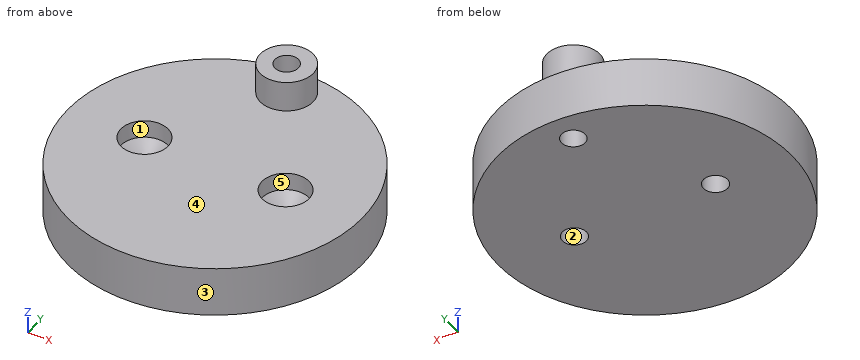
Autodesk Fusion 360 part; units mm, degrees
sketch "Esquisse1" plane through (0, 0, 0) normal (0, 0, 1) x (1, 0, 0)
  circle A0 centre (0, 0) radius 25
  circle A1 centre (-12, 0) radius 2.05
  circle A2 centre (12, 0) radius 2.05
  circle A3 centre (0, 20) radius 2
  dimension "d1" = 50
  dimension "d2" = 4.1
  dimension "d3" = 4.1
  dimension "d4" = 24
  dimension "d5" = 12
  dimension "d6" = 4
  dimension "d7" = 20
extrude "Extrusion1" add sketch "Esquisse1" along normal blind 8.5
sketch "Esquisse2" plane through (0, 0, 8.5) normal (0, 0, 1) x (-1, 0, 0)
  circle A0 centre (0, -20) radius 2
  circle A1 centre (-12, 0) radius 2.05
  circle A2 centre (12, 0) radius 2.05
  circle A3 centre (0, 0) radius 25
  circle A4 centre (0, -20) radius 4.5
  dimension "d10" = 9
extrude "Extrusion2" add sketch "Esquisse2" along normal blind 5.2 contours A4
sketch "Esquisse3" plane through (0, 0, 8.5) normal (0, 0, 1) x (-1, 0, 0)
  circle A0 centre (0, -20) radius 4.5
  circle A1 centre (-12, 0) radius 2.05
  circle A2 centre (12, 0) radius 2.05
  circle A3 centre (0, 0) radius 25
  circle A4 centre (12, 0) radius 4
  circle A5 centre (-12, 0) radius 4
  dimension "d13" = 8
  dimension "d14" = 8
extrude "Extrusion3" cut sketch "Esquisse3" against normal blind 3 contours A4 | A5
hole "Perçage1" at (-12, 0, 5.5) direction (0, 0, -1) diameter 4 depth 10 tip angle 118 countersink diameter 8 countersink angle 90
hole "Perçage2" at (12, 0, 5.5) direction (0, 0, -1) diameter 4 depth 10 tip angle 118 countersink diameter 8 countersink angle 90
The listing builds one solid part. Answer for the finished solid, in the listing's coordinates (mm). Face numbers are marked on the shaded views. A direction names the side the tool comes from. Round coordinates to 2 decimals unless told otherwise and drop trailing zeros. Write each loop counter-clockwise with the first axis right and the second up, starting at its lowest first coordinate (ties: lowest second). Pieces come first, ordered by that corner, then holes. Notation, with made-up numbers: (48, 67.25) -> (72, 67.25) arc R7 ccw to (72, 79.25) -> close; hole circle Ø11 at (-15.75, -1). An arc over 180 degrees is marked (long way). Write item = value, one per line.
1) Straight lines are drawn through the part: line 1 along Y through (x, z) = (0, 10); line 2 along Y through (x, z) = (0, 5); line 3 along Z through (x, y) = (-12.5, -17.5). For each, find the intervals that lie inside material, in ascending order. Write a range as [from, to].
Check values:
line_1 = [15.5, 18], [22, 24.5]
line_2 = [-25, 18], [22, 25]
line_3 = [0, 8.5]
2) Which of the six approach directions +Z, -Z, +X, -X, +Y, -Y give full straight-line access (tool end or side, diameter ignored) to the marked faces 1 and 2?
Check values:
face_1 = +Z
face_2 = +Z, -Z
3) For a pull along X with two mould halves and no side action, classify the marked faces 3, 4 and 5 as released by +X, released by -X, zero draft, split by the parting line, or undercut.
Check values:
face_3 = split by the parting line
face_4 = zero draft
face_5 = undercut
4) Given pin 1 (5 mm diameter, centred on x = 12.5, z = 10, fed in from +Y); pin 2 (4 mm diameter, centred on y = 3.5, z = 8, fed in from +X); pin 3 (8 mm diameter, centred on x = 12, y = 8.5, fed in from +Z), each flat-ended and moving along its own axis, determine where each tip first touches the part or whether it passes through.
Check values:
pin_1 = 22.69
pin_2 = 24.95
pin_3 = 8.5
5) Section A-A on y = 0 is taken. Write down the section's boundary in (x, z).
Check values:
outline = (-25, 0) -> (-14.05, 0) -> (-14.05, 3.55) -> (-16, 5.5) -> (-16, 8.5) -> (-25, 8.5) -> close; (-9.95, 0) -> (9.95, 0) -> (9.95, 3.55) -> (8, 5.5) -> (8, 8.5) -> (-8, 8.5) -> (-8, 5.5) -> (-9.95, 3.55) -> close; (14.05, 0) -> (25, 0) -> (25, 8.5) -> (16, 8.5) -> (16, 5.5) -> (14.05, 3.55) -> close
6) Section D-D on z = 1.25 is taken. Write down the section's boundary in (x, y), plus the area to 3 significant figures.
Check values:
outline = circle Ø50 at (0, 0); hole circle Ø4.1 at (-12, 0); hole circle Ø4 at (0, 20); hole circle Ø4.1 at (12, 0)
area = 1,920 mm²
7) Section C-C on x = -12 is taken. Write down the section's boundary in (y, z).
Check values:
outline = (-21.93, 0) -> (-2.05, 0) -> (-2.05, 3.55) -> (-4, 5.5) -> (-4, 8.5) -> (-21.93, 8.5) -> close; (2.05, 0) -> (21.93, 0) -> (21.93, 8.5) -> (4, 8.5) -> (4, 5.5) -> (2.05, 3.55) -> close
